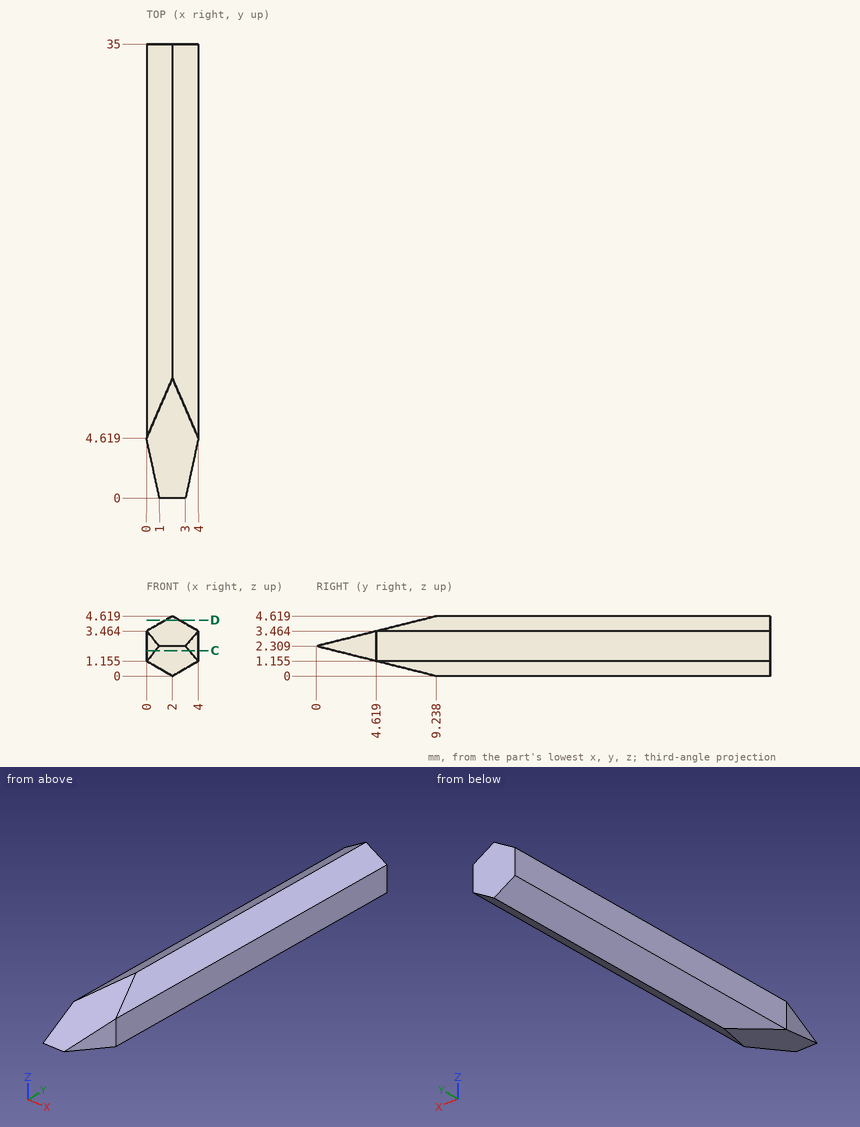
Part print with two shaded views. Sizes in mm from the minimum x, y, z corner. Give positions to 0.01 mm unless a question says otherwise; leave off trailing zeros. Order: outer loops, then holes, each group sorted by start corner. A loop starts at its lowest first (then second) coordinate and runs counter-clockwise, first axis right, second up.
1) Wall check: probe 1 along Z at (x, y) = (2.1, 26); probe 2 along Z at (x, y) = (3.55, 20) (1 decimal); probe 3 along X at (y, z) = (25.5, 3.55). Give the ranges that are in metal, low to high.
2) Saw through at C-C, the plane z = 1.95. Write the cut outline in (x, y).
3) Saw through at D-D, the plane z = 4.3. Write the cut outline in (x, y).
Computed:
1. probe 1: z = 0.06 to 4.56
1. probe 2: z = 0.9 to 3.7
1. probe 3: x = 0.15 to 3.85
2. outline: (0, 4.62) - (0.69, 1.44) - (3.31, 1.44) - (4, 4.62) - (4, 35) - (0, 35) - close
3. outline: (1.45, 7.96) - (2.55, 7.96) - (2.55, 35) - (1.45, 35) - close
